from build123d import *

# Parameters (mm, degrees)
F0_R     = 11.2
F1_DEPTH = 7


# Not quite as in the source:
# - ends of sketch curves that miss each other by under 0.0002 mm in the source are joined


with BuildPart() as f1:
    # F0 (on Front) → F1 (new body)
    with BuildSketch(Plane.XZ):
        with BuildLine():
            Line((34.3850237921, -6.6456524925), (11.9034600857, 32.216063506))
            Line((11.9034600857, 32.216063506), (10.8795652547, 33.9859719811))
            ThreePointArc((10.8795652547, 33.9859719811), (-0.5229512338, 39.7006466997), (-11.4372271683, 33.1011413973))
            ThreePointArc((-11.4372271683, 33.1011413973), (-11.443253047, 33.0906723652), (-11.449269343, 33.0801978231))
            Line((-11.449269343, 33.0801978231), (-33.8515173907, -5.7990863826))
            Line((-33.8515173907, -5.7990863826), (-34.8724977352, -7.5710060978))
            ThreePointArc((-34.8724977352, -7.5710060978), (-34.1203065589, -20.3032101841), (-22.9478157697, -26.4554889214))
            ThreePointArc((-22.9478157697, -26.4554889214), (-22.9392839252, -26.4554787883), (-22.930752089, -26.4554631407))
            Line((-22.930752089, -26.4554631407), (21.9480379364, -26.4167307195))
            Line((21.9480379364, -26.4167307195), (23.9929324806, -26.4149658832))
            ThreePointArc((23.9929324806, -26.4149658832), (34.6432297092, -19.3974365399), (34.3850237921, -6.6456524925))
        make_face()
        with Locations((-22.9592271072, -13.2554938539)):
            Circle(F0_R, mode=Mode.SUBTRACT)
        with Locations((22.9591888153, -13.2555159617)):
            Circle(F0_R, mode=Mode.SUBTRACT)
        Circle(F0_R, mode=Mode.SUBTRACT)
        with Locations((0, 26.5110097826)):
            Circle(F0_R, mode=Mode.SUBTRACT)
    extrude(amount=F1_DEPTH)


solid = f1.part
Geometry check sheet. Reference: the model listing, model coordinates, mm. Round coordinates to 2 decimals unless told otherwise and drop trailing zeros. Order: outer loops, then holes, each group sorted by start corner. A loop starts at its lowest first (then second) coordinate and runs counter-clockwise, first axis right, second up. Notation, with made-up numbers: M 31.25,23 L 36.25,23 A24 ccw 36.25,62 Z; hole C -28.5,73 d11. An arc over 180 degrees is marked long. Answer in a Markdown table with one row per item.
(1) Sectioned sample at C-C, the plane x = -19. Record the cut outline in (y, z), and give its area (3 significant figures).
Responses:
| item | result |
|---|---|
| outline | M -7,-26.45 L 0,-26.45 L 0,-23.73 L -7,-23.73 Z; M -7,-2.78 L 0,-2.78 L 0,19.98 L -7,19.98 Z |
| area | 178 mm² |
(2) Scan lines: probe 1 along Z at (x, y) = (0, -5.5); probe 2 along Z at (x, y) = (-1, -0.75); probe 3 along X at (y, z) = (-2, 31). Record each from-to range of solid material in increasing order. Write a range as from..to.
Responses:
| item | result |
|---|---|
| probe 1 | z = -26.44..-11.2, 11.2..15.31, 37.71..39.71 |
| probe 2 | z = -26.44..-11.16, 11.16..15.36, 37.67..39.67 |
| probe 3 | x = -12.65..-10.26, 10.26..12.61 |
(3) Draft check along Z on faces 1 (the face through (5.2, -7, -10.4)), 2 (the face through (34.555, -3.451, -19.562)), 3 (the face through (11.77, -3.45, -12.76)). Enter one of: released by +Z, released by -Z, zero draft, split by the parting line, or undercut.
Responses:
| item | result |
|---|---|
| face 1 | zero draft |
| face 2 | split by the parting line |
| face 3 | undercut |
(4) Go/stop test with flat-tipped pins: P1, Ø1.5, axis at x = -12, y = -5.5, coming from the +Z side; P2, Ø3, axis at y = -4.5, z = -7, coming from the +X side; P3, Ø1, axis at x = -13, y = -3, coming from the -Z side; P4, Ø6, axis at x = -14.5, z = 11, coming from the +Y side. Record where each tip stops, or that it passes through.
Responses:
| item | result |
|---|---|
| P1 | stops at z = 33.42 |
| P2 | stops at x = 35.27 |
| P3 | stops at z = -26.45 |
| P4 | stops at y = 0 |
(5) Sectioned sample at B-B, the plane x = 2. Record the cut outline in (y, z).
Responses:
| item | result |
|---|---|
| outline | M -7,-26.43 L 0,-26.43 L 0,-11.02 L -7,-11.02 Z; M -7,11.02 L 0,11.02 L 0,15.49 L -7,15.49 Z; M -7,37.53 L 0,37.53 L 0,39.56 L -7,39.56 Z |
(6) Sectioned sample at A-A, the plane z = 9. Record the cut outline in (x, y).
Responses:
| item | result |
|---|---|
| outline | M -25.32,-7 L -6.67,-7 L -6.67,0 L -25.32,0 Z; M 6.67,-7 L 25.33,-7 L 25.33,0 L 6.67,0 Z |
